Source: CAD feature listing. Evaluate the final solid. Frame: model axes, mm. Face numbers are marked on the shaded views. A direction names the side the tool comes from. Give positions to 0.01 mm unless a question says otherwise; leave off trailing zeros. Loops run counter-clockwise (first coordinate to the right, second up) from the corner with the lowest first, then second, coordinate; pieces in that order, holes last. Notation, with made-up numbers: M 19.25,3.25 L 28.25,3.25 A20 ccw 28.25,13.25 Z; hole C 24.5,-29 d11. An arc over 180 degrees is marked long. Put each result on its own line as item: value. Start each with the question number.
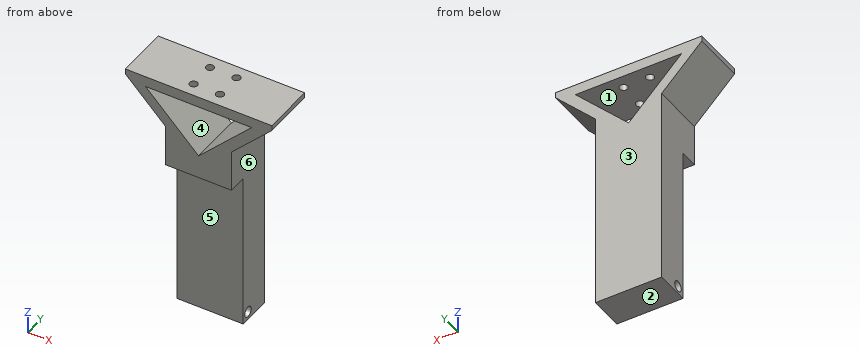
```python
from build123d import *

# Parameters (mm, degrees)
EXTRUDE_1_DEPTH     = 20
SKETCH_2_R          = 1.5
CUT_EXTRUDE_1_DEPTH = 5
SKETCH_4_W          = 24.99770673
SKETCH_4_H          = 59.73
CUT_EXTRUDE_3_DEPTH = 7
SKETCH_8_R          = 2
CUT_EXTRUDE_5_DEPTH = 41.24770673


with BuildPart() as part:
    # 스케치1 → 보스-돌출1 (new body)
    with BuildSketch(Plane(origin=(0, 0, 0), x_dir=(1, 0, 0), z_dir=(0, 1, 0))):
        Polygon((40.24770673, 92.73229327), (15.25229327, 92.73229327), (15.25229327, 17.25229327), (0, 2), (0, 0), (55.5, 0), (55.5, 2), (40.24770673, 17.25229327), align=None)
        Polygon((27.75, 24.093145751), (47.843145751, 4), (7.656854249, 4), align=None, mode=Mode.SUBTRACT)
    extrude(amount=EXTRUDE_1_DEPTH)

    # 스케치2 → 컷-돌출1 (cut)
    with BuildSketch(Plane.XY):
        with Locations((22.75, 15)):
            Circle(SKETCH_2_R)
        with Locations((32.75, 15)):
            Circle(SKETCH_2_R)
        with Locations((32.75, 5)):
            Circle(SKETCH_2_R)
        with Locations((22.75, 5)):
            Circle(SKETCH_2_R)
    extrude(amount=-CUT_EXTRUDE_1_DEPTH, mode=Mode.SUBTRACT)

    # 스케치4 → 컷-돌출3 (cut)
    with BuildSketch(Plane.XZ):
        with Locations((27.748853365, -62.86729327)):
            Rectangle(SKETCH_4_W, SKETCH_4_H)
    extrude(amount=-CUT_EXTRUDE_3_DEPTH, mode=Mode.SUBTRACT)

    # 스케치8 → 컷-돌출5 (cut, through all)
    with BuildSketch(Plane.ZY.offset(-15.25229327)):
        with Locations((-89.73229327, 10)):
            Circle(SKETCH_8_R)
    extrude(amount=-CUT_EXTRUDE_5_DEPTH, mode=Mode.SUBTRACT)


solid = part.part
```
1. Section B-B, the plane y = 15. Output: boundary loops of the cut face in (x, z).
2. Contact query for flat-ended pins moving along their axis: pin 1 (20 mm diameter, centred on x = 25, z = -50.5, fed in from -Y); pin 2 (3 mm diameter, centred on y = 4.5, z = -10.5, fed in from -X); pin 3 (12 mm diameter, centred on y = 12, z = -64.5, fed in from +X); pin 4 (2 mm diameter, centred on x = 14, z = -59, fed in from -Y). Output: stop coordinate, or through.
3. Section C-C, the plane x = 22.75. Output: boundary loops of the cut face in (y, z).
4. Ray query, line 1 (Y direction, x = 22.75, z = -2.35); line 2 (Z direction, x = 24.5, y = 11.5); line 3 (Z direction, x = 18.5, y = 11). Return the intervals inside material, ascending.
5. Section D-D, the plane z = -9. Output: boundary loops of the cut face in (x, y).
6. Set-up query: the marked faces 4, 5 and 6. Return all of +Z, -Z, +X, -X, +Y, -Y with unobstructed straight access to the full face (end or side cutting, diameter ignored); none if empty.
7. Section A-A, the plane y = 10. Output: boundary loops of the cut face in (x, z), plus the area to 3 significant figures.
8. Pull-direction query (Z, two-part tool) for the marked faces 1, 2 and 3; classes: released by +Z, released by -Z, zero draft, split by the parting line, or undercut.
Results found:
1. outline: M 0,-2 L 15.25,-17.25 L 15.25,-92.73 L 40.25,-92.73 L 40.25,-17.25 L 55.5,-2 L 55.5,0 L 34.25,0 L 34.25,-4 L 47.84,-4 L 27.75,-24.09 L 7.66,-4 L 21.25,-4 L 21.25,0 L 0,0 Z; M 24.25,-4 L 31.25,-4 L 31.25,0 L 24.25,0 Z
2. pin 1: y = 7
2. pin 2: x = 7
2. pin 3: x = 40.25
2. pin 4: through
3. outline: M 0,-33 L 7,-33 L 7,-92.73 L 20,-92.73 L 20,-19.09 L 0,-19.09 Z; M 0,-4 L 3.5,-4 L 3.5,0 L 0,0 Z; M 6.5,-4 L 13.5,-4 L 13.5,0 L 6.5,0 Z; M 16.5,-4 L 20,-4 L 20,0 L 16.5,0 Z; hole C 10,-89.73 d4
4. line 1: 0 to 3.5, 6.5 to 13.5, 16.5 to 20
4. line 2: -92.73 to -91.06, -88.41 to -20.84, -4 to 0
4. line 3: -92.73 to -91.46, -88 to -14.84, -4 to 0
5. outline: M 7,0 L 12.66,0 L 12.66,20 L 7,20 Z; M 42.84,0 L 48.5,0 L 48.5,20 L 42.84,20 Z
6. face 4: +Y, -Y
6. face 5: -Z, +X, -X, -Y
6. face 6: -Z, +X, +Y, -Y
7. outline: M 0,-2 L 15.25,-17.25 L 15.25,-87.73 L 40.25,-87.73 L 40.25,-17.25 L 55.5,-2 L 55.5,0 L 0,0 Z; M 15.25,-92.73 L 40.25,-92.73 L 40.25,-91.73 L 15.25,-91.73 Z; hole M 7.66,-4 L 27.75,-24.09 L 47.84,-4 Z
7. area: 2,110 mm²
8. face 1: undercut
8. face 2: released by -Z
8. face 3: zero draft
